from build123d import *

# Parameters (mm, degrees)
SKETCH1_W                     = 64.008
SKETCH1_H                     = 24.9936
BOSS_EXTRUDE1_DEPTH           = 6.35
SKETCH2_W                     = 64.008
SKETCH2_H                     = 6.35
BOSS_EXTRUDE2_DEPTH           = 57.15
CBORE_FOR_M5_SHCS1_AT_2_COUNT = 2
CBORE_FOR_M5_SHCS1_AT_2_PITCH = 50
SKETCH8_W                     = 6.604
SKETCH8_H                     = 6.35
CUT_EXTRUDE1_DEPTH            = 57.15
CUT_EXTRUDE2_DEPTH            = 90.374641845
CUT_EXTRUDE2_DEPTH_BACK       = 90.374641845
SKETCH9_W                     = 64.008
SKETCH9_H                     = 2.000000064


with BuildPart() as part:
    # Sketch1 → Boss-Extrude1 (new body)
    with BuildSketch(Plane.XY):
        with Locations((32.004, 12.4968)):
            Rectangle(SKETCH1_W, SKETCH1_H)
    extrude(amount=BOSS_EXTRUDE1_DEPTH)

    # Sketch2 → Boss-Extrude2 (add)
    with BuildSketch(Plane.XY.offset(6.35)):
        with Locations((32.004, 3.175)):
            Rectangle(SKETCH2_W, SKETCH2_H)
    extrude(amount=BOSS_EXTRUDE2_DEPTH)

    # Sketch7 → CBORE for M5 SHCS1 (revolve, cut)
    with BuildSketch(Plane(origin=(7, 12.5, 6.35), x_dir=(0, -1, 0), z_dir=(1, 0, 0))):
        Polygon((0, 0), (0, 6.35), (2.75, 6.35), (2.75, 5), (5, 5), (5, 0.025), (5.025, 0), align=None)
    cbore_for_m5_shcs1 = revolve(axis=Axis((7, 12.5, 12.7), (0, 0, -1)), mode=Mode.SUBTRACT)

    # CBORE for M5 SHCS1 at 2: CBORE for M5 SHCS1 ×2
    with Locations(*[(i * CBORE_FOR_M5_SHCS1_AT_2_PITCH, 0, 0) for i in range(1, CBORE_FOR_M5_SHCS1_AT_2_COUNT)]):
        add(cbore_for_m5_shcs1, mode=Mode.SUBTRACT)

    # Sketch8 → Cut-Extrude1 (cut)
    with BuildSketch(Plane.XY.offset(63.5)):
        with Locations((3.302, 3.175)):
            Rectangle(SKETCH8_W, SKETCH8_H)
        with Locations((60.706, 3.175)):
            Rectangle(SKETCH8_W, SKETCH8_H)
    extrude(amount=-CUT_EXTRUDE1_DEPTH, mode=Mode.SUBTRACT)

    # Sketch9 → Cut-Extrude2 (cut, two sides: drawn at the far end of the back side and taken through both)
    with BuildSketch(Plane.XY.offset(6.35).offset(-CUT_EXTRUDE2_DEPTH_BACK)):
        with Locations((32.004, 1.000000032)):
            Rectangle(SKETCH9_W, SKETCH9_H)
    extrude(amount=CUT_EXTRUDE2_DEPTH + CUT_EXTRUDE2_DEPTH_BACK, mode=Mode.SUBTRACT)


solid = part.part
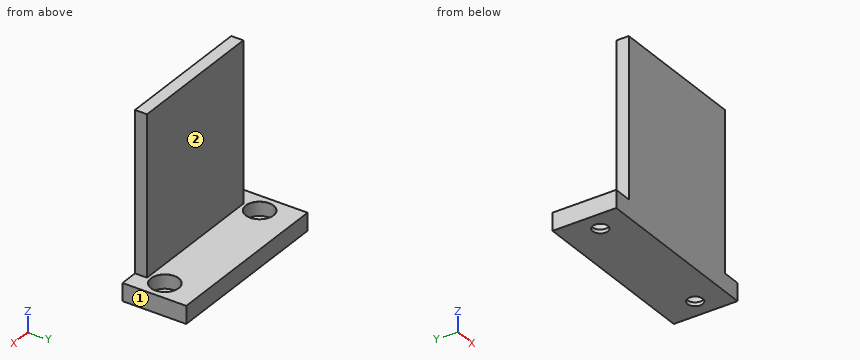
Input: part model. Units: mm. Frame: model coordinates. Face numbers are marked on the shaded views. A direction names the side the tool comes from. Round coordinates to 2 decimals unless told otherwise and drop trailing zeros. Loops run counter-clockwise (first coordinate to the right, second up) from the corner with the lowest first, then second, coordinate; pieces in that order, holes last. Notation, with made-up numbers: (19.5, -33.75) -> (54.5, -33.75) arc R33 cw to (54.5, 3.25) -> close; hole circle Ø3 at (49.25, -13). An arc over 180 degrees is marked (long way). Answer as a JSON object with one key per item and string values. Group by question number.
1) Section query A-A on y = 12.5. Output: boundary loops of the cut face in (x, z) (3 decimals).
2) Pin query (flat end, axial travel): pin 1 (11.5 mm diameter, centred on x = 7, y = 12.5, fed in from +Z); pin 2 (6.5 mm diameter, centred on x = 7, y = 12.5, fed in from +Z); pin 3 (1 mm diameter, centred on x = 51.5, y = 13.5, fed in from +Z); pin 4 (4.5 mm diameter, centred on x = 57, y = 12.5, fed in from -Z). Return the tip coordinate at first contact, or that it passes through.
3) Section query D-D on z = 39. Output: boundary loops of the cut face in (x, y), plus the area to 3 significant figures.
4) Section query C-C on x = 27. Output: boundary loops of the cut face in (y, z), plus the area to 3 significant figures.
5) Reachability of the marked faces 1 and 2 from +Z, -Z, +X, -X, +Y, -Y: full face, straight path, thin tool, end or side. Return the list, or none.
6) Ray query, L1, parallel to X at y = 12.5, z = 4.5; L2, parallel to X at y = 12.5, z = 0.9; L3, parallel to Y at x = 7, z = 0.75. Return the intervals inside material, ascending.
7) Section query B-B on y = 5. Output: boundary loops of the cut face in (x, z), plus the area to 3 significant figures.
Reply:
{
 "1": {"outline": "(0, 0) -> (4.25, 0) -> (4.25, 1.35) -> (2, 1.35) -> (2, 6.325) -> (1.975, 6.35) -> (0, 6.35) -> close; (9.75, 0) -> (54.25, 0) -> (54.25, 1.35) -> (52, 1.35) -> (52, 6.325) -> (51.975, 6.35) -> (12.025, 6.35) -> (12, 6.325) -> (12, 1.35) -> (9.75, 1.35) -> close; (59.75, 0) -> (64.008, 0) -> (64.008, 6.35) -> (62.025, 6.35) -> (62, 6.325) -> (62, 1.35) -> (59.75, 1.35) -> close"},
 "2": {"pin 1": "stops at z = 6.35", "pin 2": "stops at z = 1.35", "pin 3": "stops at z = 6.35", "pin 4": "passes through"},
 "3": {"outline": "(6.6, 2) -> (57.4, 2) -> (57.4, 6.35) -> (6.6, 6.35) -> close", "area": "221 mm2"},
 "4": {"outline": "(2, 0) -> (24.99, 0) -> (24.99, 6.35) -> (6.35, 6.35) -> (6.35, 63.5) -> (2, 63.5) -> close", "area": "395 mm2"},
 "5": {"face 1": "+Z, -Z, +X, +Y, -Y", "face 2": "+Z, +X, -X, +Y"},
 "6": {"L1": "x = 0 to 2, 12 to 52, 62 to 64.01", "L2": "x = 0 to 4.25, 9.75 to 54.25, 59.75 to 64.01", "L3": "y = 2 to 9.75, 15.25 to 24.99"},
 "7": {"outline": "(0, 0) -> (64.01, 0) -> (64.01, 6.35) -> (57.4, 6.35) -> (57.4, 63.5) -> (6.6, 63.5) -> (6.6, 6.35) -> (0, 6.35) -> close", "area": "3,310 mm2"}
}
